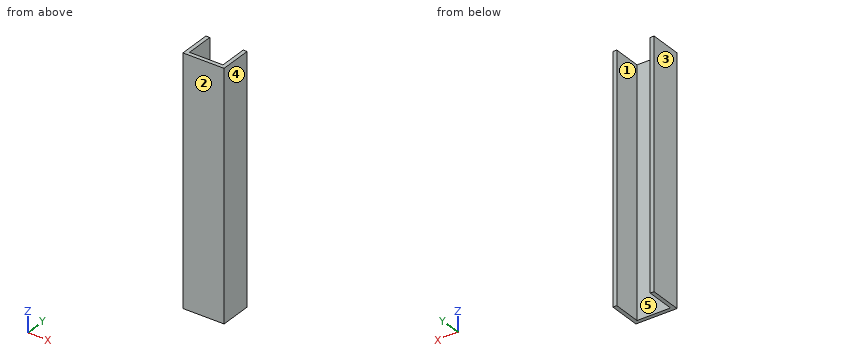
Autodesk Inventor part; units mm, degrees
ref_plane "YZ Plane" through (0, 0, 0) normal (1, 0, 0) x (0, 1, 0)
ref_plane "XZ Plane" through (0, 0, 0) normal (0, 1, 0) x (-1, 0, 0)
ref_plane "XY Plane" through (0, 0, 0) normal (0, 0, 1) x (1, 0, 0)
sketch "Sketch1" plane through (0, 0, 0) normal (0, 0, 1) x (1, 0, 0)
  line L0 (-16, -12.5) -> (16, -12.5)
  line L1 (16, -12.5) -> (16, 12.5)
  line L2 (16, 12.5) -> (13, 12.5)
  line L3 (13, 12.5) -> (13, -9.5)
  line L4 (13, -9.5) -> (-13, -9.5)
  line L5 (-13, -9.5) -> (-13, 12.5)
  line L6 (-13, 12.5) -> (-16, 12.5)
  line L7 (-16, 12.5) -> (-16, -12.5)
  point P0 (0, 0)
  dimension "d0" = 32
  dimension "d1" = 25
  dimension "d2" = 3
  dimension "d3" = 90
  dimension "d4" = 22
  dimension "d5" = 26
  dimension "d6" = 22
  dimension "d7" = 3
  dimension "d8" = 25
  dimension "d10" = 12.5
  dimension "d11" = 16
extrude "Extrusion1" add sketch "Sketch1" against normal blind 190
equation "\"d5\" = d0 - 2 * d7"
properties part number "Chassis Vertical"
The model under review builds one solid part; all positions refer to its coordinate system, in mm. Face numbers are marked on the shaded views. A direction names the side the tool comes from. Coordinates: 2 decimals unless noted, no trailing zeros. Write each loop counter-clockwise with the first axis right and the second up, starting at its lowest first coordinate (ties: lowest second). Pieces come first, ordered by that corner, then holes. Notation, with made-up numbers: (20.5, 49) - (46.5, 49) arc R23 ccw to (46.5, 62) - close; hole circle Ø10 at (26.25, 88). An arc over 180 degrees is marked (long way). Answer in a Markdown table with one row per item. Add a question column.
Q1. For the marked faces 4 and 5, list the 3-axis set-ups (+Z, -Z, +X, -X, +Y, -Y) from which the entire face can be reached by the end or side of a thin tool; tool diameter is ignored.
Q2. Consider section B-B on z = -60.5. Give the boundary of the cut face in (x, y), then the cut area to 3 significant figures.
Q3. Consider section A-A on y = -7.75. Give the boundary of the cut face in (x, z), then the cut area to 3 significant figures.
Q4. Draft analysis for pull direction X (two halves, no side actions). For the marked faces 1, 2 and 3, state which applies: +X half, -X half, draft (parallel to the pull), parting line (faces both ways), or undercut.
Q5. Clearance check with flat-ended pins moving along their axes: pin 1 (5 mm diameter, centred on x = -3, y = -8, fed in from -Z); pin 2 (13 mm diameter, centred on x = -4.5, z = -69, fed in from +Y). State where each tip first meets the part, or that it passes through.
Q6. Consider section C-C on x = 5. Give the boundary of the cut face in (y, z).
Q7. To check wall thickness, follow line 1 along X through (y, z) = (3.25, -23); line 2 along Y through (x, z) = (-10, -146). State the ranges of each line that lie inside material, in increasing order. Write a range as from..to.
Answers below:
| question | item | result |
|---|---|---|
| 1 | face 4 | +Z, -Z, +X, +Y, -Y |
| 1 | face 5 | +Z, -Z, +Y |
| 2 | outline | (-16, -12.5) - (16, -12.5) - (16, 12.5) - (13, 12.5) - (13, -9.5) - (-13, -9.5) - (-13, 12.5) - (-16, 12.5) - close |
| 2 | area | 228 mm² |
| 3 | outline | (-16, -190) - (-13, -190) - (-13, 0) - (-16, 0) - close; (13, -190) - (16, -190) - (16, 0) - (13, 0) - close |
| 3 | area | 1,140 mm² |
| 4 | face 1 | undercut |
| 4 | face 2 | draft |
| 4 | face 3 | -X half |
| 5 | pin 1 | z = -190 |
| 5 | pin 2 | y = -9.5 |
| 6 | outline | (-12.5, -190) - (-9.5, -190) - (-9.5, 0) - (-12.5, 0) - close |
| 7 | line 1 | -16..-13, 13..16 |
| 7 | line 2 | -12.5..-9.5 |
